CAD build for the part. Positions are in the model's coordinates, mm. A direction names the side the tool comes from. Coordinates: 2 decimals unless noted, no trailing zeros. Loops run counter-clockwise (first coordinate to the right, second up) from the corner with the lowest first, then second, coordinate; pieces in that order, holes last. Notation, with made-up numbers: (-34, 60.5) -> (17, 60.5) arc R33 cw to (17, 88.5) -> close; hole circle Ø10 at (21, 54.5). An arc over 180 degrees is marked (long way). Write each question's results on one line, items separated by ' | '.
```python
from build123d import *

# Parameters (mm, degrees)
F0_W     = 31.75
F0_H     = 27.94
F2_R     = 3.81
F3_DEPTH = 70.2046528459
F4_T     = -5.08


with BuildPart() as f1:
    # F0 (on Front) → F1 (revolve)
    with BuildSketch(Plane.XZ):
        with Locations((-0.1187622547, 17.9933030483)):
            Rectangle(F0_W, F0_H)
    revolve(axis=Axis((15.7562377453, 0, 17.9933030483), (0, 0, -1)))

    # F2 (on face) → F3 (cut)
    with BuildSketch(Plane.XY.offset(31.9633030483)):
        with Locations((15.7562377453, 0)):
            Circle(F2_R)
    extrude(amount=-F3_DEPTH, mode=Mode.SUBTRACT)

    # F4
    f4_openings = [f1.faces().sort_by_distance(p)[0] for p in [
        (47.506238, 0, 17.993303),
    ]]
    offset(amount=F4_T, openings=f4_openings)


solid = f1.part
```
Q1. Cut at D-D on y = 27. Write the cut outline in (x, z).
Results are:
outline: (-0.95, 4.02) -> (32.46, 4.02) -> (32.46, 9.1) -> (-0.95, 9.1) -> close; (-0.95, 26.88) -> (32.46, 26.88) -> (32.46, 31.96) -> (-0.95, 31.96) -> close
Q2. Cut at B-B on x = 38. Write the cut outline in (y, z), and give its area (3 significant figures).
Results are:
outline: (-22.66, 4.02) -> (22.66, 4.02) -> (22.66, 9.1) -> (-22.66, 9.1) -> close; (-22.66, 26.88) -> (22.66, 26.88) -> (22.66, 31.96) -> (-22.66, 31.96) -> close | area: 460 mm^2
Q3. Which spindle directions (+Z, -Z, +X, -X, +Y, -Y) get a long thin tool onto all of the face, cutting with end or side? Do faces 4 (the cylindrical face through (40.95, -19.32, 29.46)), 5 (the flat face through (9, -7, 9.103)). Say none if no direction does.
Results are:
face 4: +Z, -Z | face 5: none
Q4. Pull direction Z, two halves, no side cores. Call faces 1 (the cylindrical face through (23.97, -3.4, 18.12)), 2 (the flat face through (9, 0, 31.963)), 3 (the cylindrical face through (40.95, -19.32, 6.6)): +Z half, -Z half, draft (parallel to the pull), parting line (faces both ways), or undercut.
Results are:
face 1: undercut | face 2: +Z half | face 3: draft
Q5. Cut at C-C on z = 7. Write the cut outline in (x, y), and give its area (3 significant figures).
Results are:
outline: circle Ø63.5 at (15.76, 0); hole circle Ø7.62 at (15.76, 0) | area: 3,120 mm^2
Q6. Drop flat-ended pins along their axis: pin 1 (6 mm diameter, centred on y = -8, z = 22, fed in from -X); pin 2 (2 mm diameter, centred on x = 20.5, z = 19.5, fed in from -Y); pin 3 (1.5 mm diameter, centred on y = -10.5, z = 15, fed in from +X); pin 4 (3 mm diameter, centred on y = 4, z = 13, fed in from +X). Give the stop position or say it passes through.
Results are:
pin 1: x = 8.41 | pin 2: y = -8.06 | pin 3: through | pin 4: x = 24.29
Q7. Cut at A-A on y = 0. Write the cut outline in (x, z).
Results are:
outline: (-15.99, 4.02) -> (11.95, 4.02) -> (11.95, 31.96) -> (-15.99, 31.96) -> (-15.99, 26.88) -> (6.87, 26.88) -> (6.87, 9.1) -> (-15.99, 9.1) -> close; (19.57, 4.02) -> (47.51, 4.02) -> (47.51, 9.1) -> (24.65, 9.1) -> (24.65, 26.88) -> (47.51, 26.88) -> (47.51, 31.96) -> (19.57, 31.96) -> close
Q8. Wall check: L1, parallel to Z at x = 10, y = 21; L2, parallel to Y at x = 21, z = 20.75; L3, parallel to Y at x = 8, z = 20. Give the ranges that are in metal, low to high. Write a range as from..to.
Results are:
L1: 4.02..9.1, 26.88..31.96 | L2: -7.18..7.18 | L3: -4.34..4.34
